```python
from build123d import *

# Parameters (mm, degrees)
SWEEP1_PROFILE_R   = 2.5
SKETCH14_R         = 1.5
CUT_EXTRUDE1_DEPTH = 4


with BuildPart() as part:
    # Sweep1: sweep along a path in Sketch1
    with BuildLine(Plane(origin=(0, 0, 0), x_dir=(1, 0, 0), z_dir=(0, 1, 0))) as sweep1_path:
        ThreePointArc((-10, 0), (0, 10), (10, 0))
    # Sweep1 profile (on start of the path) → Sweep1 (sweep)
    with BuildSketch(Plane(origin=(-10, 0, 0), x_dir=(-1, 0, 0), z_dir=(0, 0, -1))):
        Circle(SWEEP1_PROFILE_R)
    sweep(path=sweep1_path.line)

    # Sketch14 → Cut-Extrude1 (cut)
    with BuildSketch(Plane.XY):
        with Locations((-10, 0)):
            Circle(SKETCH14_R)
    cut_extrude1 = extrude(amount=-CUT_EXTRUDE1_DEPTH, mode=Mode.SUBTRACT)

    # Mirror1: Cut-Extrude1 across plane
    add(cut_extrude1.mirror(Plane(origin=(0, 0, 0), x_dir=(0, 0, 1), z_dir=(1, 0, 0))), mode=Mode.SUBTRACT)


solid = part.part
```
The listing builds one solid part. Answer for the finished solid, in the listing's coordinates (mm). A direction names the side the tool comes from. Round coordinates to 2 decimals unless told otherwise and drop trailing zeros. Order: outer loops, then holes, each group sorted by start corner. A loop starts at its lowest first (then second) coordinate and runs counter-clockwise, first axis right, second up. Notation, with made-up numbers: (-32.5, 84.25) - (-23.5, 84.25) arc R25 cw to (-23.5, 99.25) - close; hole circle Ø6 at (38, 67). An arc over 180 degrees is marked (long way). Put each result on its own line as item: value. Start each with the question number.
(1) Given P1, Ø3, axis at y = -1.5, z = -9.5, coming from the -X side; P2, Ø3, axis at x = -0.5, y = 0.5, coming from the +Z side; P3, Ø1.5, axis at y = -1, z = -8, coming from the +X side, each flat-ended and moving along its own axis, determine where each tip first touches the part or whether it passes through.
(2) Straight lines are drawn through the part: probe 1 along Y at (x, z) = (10, -0.95); probe 2 along X at (y, z) = (0.75, -3.75); probe 3 along X at (y, z) = (0.35, -5.5). For each, find the intervals that lie inside material, in ascending order. Write a range as from..to.
(3) Find section B-B (z = -2.75). State how many separate pieces and enclosed holes the cut face has, plus the area to 3 significant figures.
(4) For faces 1 (the flat face through (10, 0, -4)), 2 (the flat face through (-10, -2, 0)), determine the directions among +Z, -Z, +X, -X, +Y, -Y from which every point of the face is accessible in a straight line to the end or side of a thin tool.
(5) Find section A-A (y = 0). Give the vertices of the cut face in (x, z), plus the area to 3 significant figures.
(6) Determine the mould class of faces 3 (the cylindrical face through (11.5, 0.07, -1.97)), 4 (the flat face through (10, -2, 0)) for opening direction Y: released by +Y, released by -Y, zero draft, split by the parting line, or undercut.
Reply:
1. P1: x = -9.28
1. P2: z = -7.24
1. P3: x = 10.01
2. probe 1: -2.5..-1.5, 1.5..2.5
2. probe 2: -11.8..-11.3, -8.7..-6.63, 6.63..8.7, 11.3..11.8
2. probe 3: -11.2..-5.14, 5.14..11.2
3. separate pieces: 2
3. enclosed holes: 2
3. area: 26.8 mm^2
4. face 1: +Z
4. face 2: +Z, +X, -X, +Y, -Y
5. outline: (-12.5, 0) arc R12.5 ccw to (12.5, 0) - (11.5, 0) - (11.5, -4) - (8.5, -4) - (8.5, 0) - (7.5, 0) arc R7.5 cw to (-7.5, 0) - (-8.5, 0) - (-8.5, -4) - (-11.5, -4) - (-11.5, 0) - close
5. area: 133 mm^2
6. face 3: undercut
6. face 4: zero draft
